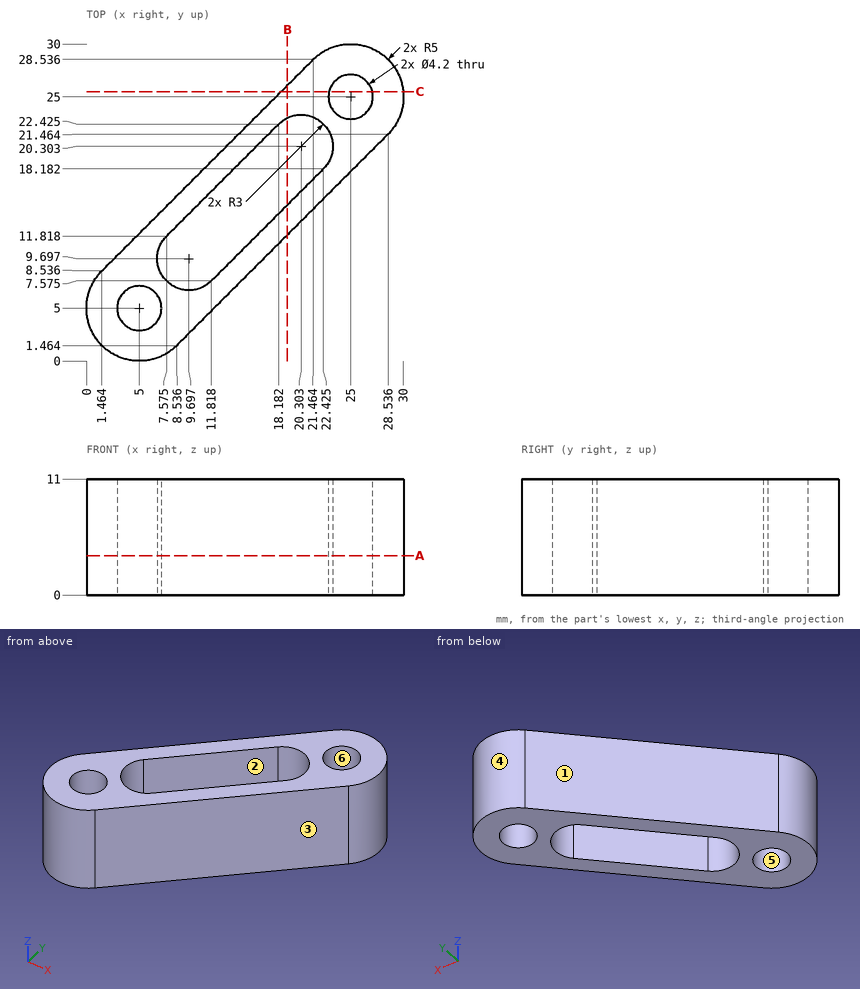
Answer from the drawing. Dimensions are ordinates in mm from the lowest x, y and z of the part. A direction names the side the tool comes from. Coordinates: 2 decimals unless noted, no trailing zeros. Loops run counter-clockwise (first coordinate to the right, second up) from the corner with the lowest first, then second, coordinate; pieces in that order, holes last.
1) For the marked faces 1 and 2, determine the directions among +Z, -Z, +X, -X, +Y, -Y from which every point of the face is accessible in a straight line to the end or side of a thin tool.
Results:
face 1: +Z, -Z, -X, +Y
face 2: +Z, -Z
2) Section B-B (x = 19) is taken. Give the vertices of the cut face in (y, z) (1 decimal).
Results:
outline: (11.9, 0) - (14.8, 0) - (14.8, 11) - (11.9, 11) - close; (23, 0) - (26.1, 0) - (26.1, 11) - (23, 11) - close
3) Flat-ended cylindrical pins translate along their axes: pin 1 (4 mm diameter, centred on x = 5, y = 5, fed in from +Z) (3 decimals); pin 2 (6 mm diameter, centred on x = 18, z = 3.5, fed in from +Y); pin 3 (6 mm diameter, centred on y = 7, z = 1.5, fed in from +X). Find the tip coordinate at first contact, or state that the pin passes through.
Results:
pin 1: passes through
pin 2: stops at y = 28.07
pin 3: stops at x = 17.07
4) Section A-A (z = 3.75) is taken. Give the vertices of the cut face in (x, y) (1 decimal).
Results:
outline: (1.5, 8.5) arc R5 ccw to (8.5, 1.5) - (28.5, 21.5) arc R5 ccw to (21.5, 28.5) - close; hole circle Ø4.2 at (5, 5); hole (7.6, 11.8) arc R3 ccw to (11.8, 7.6) - (22.4, 18.2) arc R3 ccw to (18.2, 22.4) - close; hole circle Ø4.2 at (25, 25)
5) For a pull along Y with two mould halves and no side action, classify the marked faces 3, 4, 5 and 6 as +Y half, -Y half, draft (parallel to the pull), parting line (faces both ways), or undercut.
Results:
face 3: -Y half
face 4: parting line
face 5: undercut
face 6: undercut
6) Consider probe 1 along X at (y, z) = (22.5, 10) (1 decimal); probe 2 along Y at (x, z) = (5, 8.25); probe 3 along Y at (x, z) = (21.5, 10.5) (1 decimal). Determine where each line is inside the solid, lowest interval first.
Results:
probe 1: x = 15.4 to 18.3, 22.3 to 29.3
probe 2: y = 0 to 2.9, 7.1 to 12.07
probe 3: y = 14.4 to 17.3, 23.1 to 28.6
7) Section C-C (y = 25.5) is taken. Give the vertices of the cut face in (x, z) (1 decimal).
Results:
outline: (18.4, 0) - (23, 0) - (23, 11) - (18.4, 11) - close; (27, 0) - (30, 0) - (30, 11) - (27, 11) - close
